Geometry: final body of the model. Coordinates: model frame, mm. A direction names the side the tool comes from. Round coordinates to 2 decimals unless told otherwise and drop trailing zeros. Write each loop counter-clockwise with the first axis right and the second up, starting at its lowest first coordinate (ties: lowest second). Pieces come first, ordered by that corner, then holes. Notation, with made-up numbers: (66, 58.25) - (114, 58.25) arc R4 ccw to (114, 62.25) - close; hole circle Ø4 at (56, -9.75). An arc over 180 degrees is marked (long way). Write each question's results on one line, items separated by ' | '.
Autodesk Fusion 360 part; units mm, degrees
sketch "Sketch1" plane through (0, 0, 0) normal (1, 0, 0) x (0, 1, 0)
  circle A0 centre (0, 0) radius 3.58
  circle A1 centre (14, 0) radius 2
  line L0 (0.404, 3.5571) -> (14.2257, 1.9872)
  line L1 (0.404, -3.5571) -> (14.2257, -1.9872)
  circle A2 centre (14, 0) radius 0.5
  circle A3 centre (12, 0) radius 0.5
  circle A4 centre (10, 0) radius 0.5
  circle A5 centre (8, 0) radius 0.5
  circle A6 centre (6, 0) radius 0.5
  line L2 (0, 7) -> (0, -7.5)
  circle A7 centre (-6, 0) radius 0.5
  circle A8 centre (-8, 0) radius 0.5
  line L3 (-0.404, 3.5571) -> (-14.2257, 1.9872)
  circle A9 centre (-10, 0) radius 0.5
  circle A10 centre (-12, 0) radius 0.5
  circle A11 centre (-14, 0) radius 2
  circle A12 centre (-14, 0) radius 0.5
  line L4 (-0.404, -3.5571) -> (-14.2257, -1.9872)
  dimension "d4" = 7.16
  dimension "d5" = 4
  dimension "d6" = 14
  dimension "d7" = 1
  dimension "d10" = -8
  dimension "d11" = 0
extrude "Extrude1" add sketch "Sketch1" along normal blind 1.8 contours A0 L2 | A0 A1 L0 L1 A3 | A0 L2 | A1 A3 | A0 L3 A10 A11 L4 | A10 A11 picked at (12.8171, -0.6045) picked at (-12.8171, -0.6045) makes body 1
extrude "Extrude2" add sketch "Sketch1" along normal blind 1.8 separate body contours A0 L2 | A0 A1 L0 L1 A3 | A0 L2 | A1 A3 picked at (12.8171, -0.6045) makes body 2
sketch "Sketch2" plane through (0, 0, 0) normal (1, 0, 0) x (0, 1, 0)
extrude "Extrude3" add sketch "Sketch1" against normal blind 1.83 contours A0 L2 | A0 L2 bodies 1
sketch "Sketch3" plane through (1.8, 0, 0) normal (1, 0, 0) x (0, 1, 0)
  circle A0 centre (-8, 0) radius 0.5
  circle A1 centre (8, 0) radius 0.5
  circle A2 centre (-10, 0) radius 0.5
  circle A3 centre (10, 0) radius 0.5
  circle A4 centre (-6, 0) radius 0.5
  circle A5 centre (14, 0) radius 0.5
  circle A6 centre (-14, 0) radius 0.5
  circle A7 centre (12, 0) radius 0.5
  circle A8 centre (6, 0) radius 0.5
  circle A9 centre (-12, 0) radius 0.5
  line L0 (0.404, -3.5571) -> (14.2257, -1.9872)
  arc A10 (14.2257, -1.9872) -> (14.2257, 1.9872) centre (14, 0) ccw
  line L1 (14.2257, 1.9872) -> (0.404, 3.5571)
  arc A11 (0.404, 3.5571) -> (-0.404, 3.5571) centre (0, 0) ccw
  line L2 (-0.404, 3.5571) -> (-14.2257, 1.9872)
  arc A12 (-14.2257, 1.9872) -> (-14.2257, -1.9872) centre (-14, 0) ccw
  line L3 (-14.2257, -1.9872) -> (-0.404, -3.5571)
  arc A13 (-0.404, -3.5571) -> (0.404, -3.5571) centre (0, 0) ccw
  circle A14 centre (0, 0) radius 2.5
  circle A15 centre (0, 0) radius 3.58
  dimension "d18" = 5
extrude "Extrude4" cut sketch "Sketch3" against normal blind 0.8 contours A14 bodies 1
sketch "Sketch4" plane through (1, 0, 0) normal (1, 0, 0) x (0, 1, 0)
  circle A0 centre (0, 0) radius 2.5
  circle A1 centre (0, 0) radius 2.5
  circle A2 centre (0, 0) radius 1
  dimension "d21" = 2
extrude "Extrude5" cut sketch "Sketch4" against normal blind 13.5 contours A2 bodies 1
sketch "Sketch5" plane through (-1.83, 0, 0) normal (-1, 0, 0) x (0, -1, 0)
  circle A0 centre (0, 0) radius 1
  circle A1 centre (0, 0) radius 3.58
  circle A2 centre (0, 0) radius 2.3
  dimension "d24" = 4.6
extrude "Extrude6" cut sketch "Sketch5" against normal blind 1.5 contours A2 bodies 1
extrude "Extrude7" add sketch "Sketch1" against normal blind 1.83 contours A0 L2 | A0 L2 bodies 2
extrude "Extrude8" cut sketch "Sketch3" against normal blind 0.8 contours A14 bodies 2
extrude "Extrude9" cut sketch "Sketch5" against normal blind 1.5 contours A2 bodies 2
extrude "Extrude10" cut 1 faces at (-1.83, 0.6188, -0.2429) along direction (1, 0, 0) blind 27.5 on bodies 2 bodies 2
hidden bodies 2
equation "d4 = 3.58 * 2 mm"
equation "d16 = -3.43 mm + 1.6 mm"
equation "d27 = -3.43 mm + 1.6 mm"
Q1. Ray query, line 1 along X through (y, z) = (4, 1); line 2 along Z through (x, y) = (0.4, 6); line 3 along Y through (x, z) = (-1.4, 0.5) (3 decimals). Return the intervals inside material, ascending.
Answer block:
line 1: 0 to 1.8 | line 2: -2.92 to -0.5, 0.5 to 2.92 | line 3: -3.545 to -2.245, 2.245 to 3.545
Q2. Access query for faces 4 (the cylindrical face through (0.887, -7.523, -0.15)), 5 (the flat face through (1, 1, -1)), 6 (the cylindrical face through (-0.85, -0.47, -3.55)). Directions: +Z, -Z, +X, -X, +Y, -Y. A direction counts if a zero-diameter tool reaches every point of the face in a straight line with its end or side. Return the directions, or none.
Answer block:
face 4: +X, -X | face 5: +X | face 6: -X
Q3. Section query D-D, the plane y = -3. Return loops of the section in (x, z).
Answer block:
outline: (-1.83, -1.95) - (0, -1.95) - (0, -3.26) - (1.8, -3.26) - (1.8, 3.26) - (0, 3.26) - (0, 1.95) - (-1.83, 1.95) - close
Q4. Pin query (flat end, axial travel): pin 1 (1.5 mm diameter, centred on x = 1.5, y = -11, fed in from +Z); pin 2 (1.5 mm diameter, centred on x = 0.5, y = 3, fed in from -Z); pin 3 (1.5 mm diameter, centred on y = -1, z = 0.5, fed in from +X). Return the tip coordinate at first contact, or that it passes through.
Answer block:
pin 1: z = 2.44 | pin 2: z = -3.35 | pin 3: x = 1
Q5. Mould query, pull axis Y, two halves, no side actions, for faces 1 (the cylindrical face through (0.9, -12.5, 0)), 2 (the flat face through (1.8, 0, -3)), 3 (the flat face through (0.887, -7.218, 2.783)). Classes: pulls with the +Y half, pulls with the -Y half, needs draft (parallel to the pull), parting line crosses it, or undercut.
Answer block:
face 1: undercut | face 2: needs draft | face 3: pulls with the -Y half
Q6. Section query A-A, the plane x = 0.4. Give the number of separate pieces and of enclosed holes in the cut face, plus the area to 3 significant figures.
Answer block:
separate pieces: 1 | enclosed holes: 11 | area: 159 mm2
Q7. Section query B-B, the plane y = -12. Return loops of the section in (x, z), plus the area to 3 significant figures.
Answer block:
outline: (0, -2.24) - (1.8, -2.24) - (1.8, -0.5) - (0, -0.5) - close; (0, 0.5) - (1.8, 0.5) - (1.8, 2.24) - (0, 2.24) - close | area: 6.26 mm2
